Can you work these out from the drawing? Everything is in mm from the part's minimum corner. A direction names the side the tool comes from. Round coordinates to 2 decimals unless told otherwise and drop trailing zeros. Loops run counter-clockwise (first coordinate to the right, second up) from the corner with the lowest first, then second, coordinate; pieces in that order, holes last. Notation, with made-up numbers: M 75,9 L 100,9 A25 ccw 100,40 Z; hole C 44.5,-35 d11. An arc over 180 degrees is marked long. Use a Markdown table: item, result.
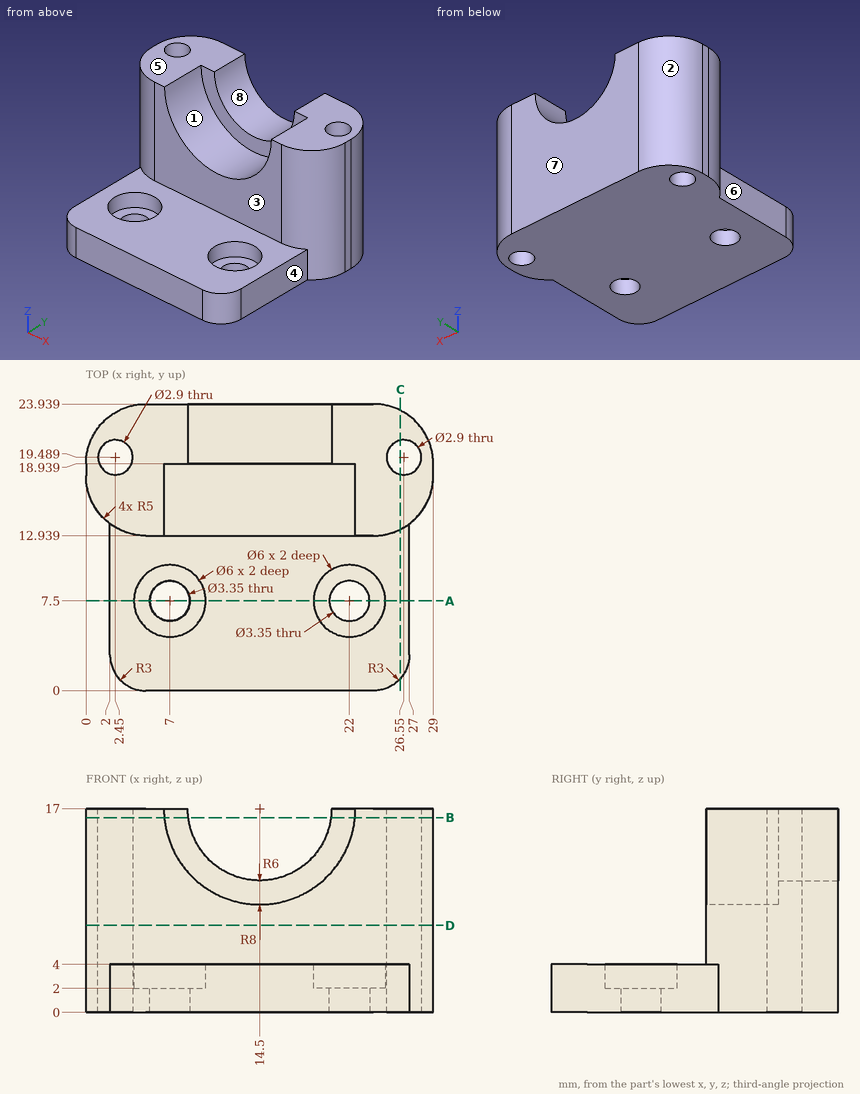
Q1. Imagine slicing it at A-A, the plane y = 7.5. Please give me the cut outline in (x, z) (1 decimal).
Return value:
| item | result |
|---|---|
| outline | M 2,0 L 5.3,0 L 5.3,2 L 4,2 L 4,4 L 2,4 Z; M 8.7,0 L 20.3,0 L 20.3,2 L 19,2 L 19,4 L 10,4 L 10,2 L 8.7,2 Z; M 23.7,0 L 27,0 L 27,4 L 25,4 L 25,2 L 23.7,2 Z |
Q2. I need wall thicknesses on line 1 (Y direction, x = 7, z = 3.35); line 2 (Y direction, x = 22, z = 0.5) (1 decimal); line 3 (Z direction, x = 3.25, y = 2.75). Which ranges of each line are inside material? Lowest first, please. Write a range as from..to.
Return value:
| item | result |
|---|---|
| line 1 | y = 0..4.5, 10.5..23.94 |
| line 2 | y = 0..5.8, 9.2..23.9 |
| line 3 | z = 0..4 |
Q3. Imagine slicing it at D-D, the plane z = 7.25. Please give me the cut outline in (x, y).
Return value:
| item | result |
|---|---|
| outline | M 0,17.94 A5 ccw 5,12.94 L 24,12.94 A5 ccw 29,17.94 L 29,18.94 A5 ccw 24,23.94 L 5,23.94 A5 ccw 0,18.94 Z; hole C 2.45,19.49 d2.9; hole C 26.55,19.49 d2.9 |
Q4. Will these pins go through, and if not, where does the flat tip stop? P1, Ø3, axis at y = 8.5, z = 2, coming from the +X side; P2, Ø4.5, axis at y = 10.5, z = 3, coming from the -X side; P3, Ø9, axis at x = 13, z = 15, coming from the -Y side.
Return value:
| item | result |
|---|---|
| P1 | stops at x = 27 |
| P2 | stops at x = 2 |
| P3 | stops at y = 18.94 |
Q5. Imagine slicing it at B-B, the plane z = 16.25. Give the number of separate pieces and of enclosed holes in the cut face, then the cut area to 3 significant figures.
Return value:
| item | result |
|---|---|
| separate pieces | 2 |
| enclosed holes | 2 |
| area | 129 mm^2 |
Q6. We'd pull the mould along X, two halves only. Please class the marked faces 6, 7 and 8: pulls with the +X half, pulls with the -X half, needs draft (parallel to the pull), parting line crosses it, or undercut.
Return value:
| item | result |
|---|---|
| face 6 | pulls with the -X half |
| face 7 | needs draft |
| face 8 | undercut |
Q7. Imagine slicing it at C-C, the plane x = 26.25. Please give me the cut outline in (y, z) (1 decimal).
Return value:
| item | result |
|---|---|
| outline | M 1,0 L 18.1,0 L 18.1,17 L 13.5,17 L 13.5,4 L 1,4 Z; M 20.9,0 L 23.4,0 L 23.4,17 L 20.9,17 Z |
Q8. For the marked faces 1, 2, 3, 4 and 5, which set-ups out of +Z, -Z, +X, -X, +Y, -Y let a thin tool reach every point of the face, with its end or its side?
Return value:
| item | result |
|---|---|
| face 1 | +Z, -Y |
| face 2 | +Z, -Z, -X, +Y |
| face 3 | +Z, +X, -X, -Y |
| face 4 | +Z, -Z, +X, -Y |
| face 5 | +Z, +X, -X, +Y, -Y |
